```python
from build123d import *

# Parameters (mm, degrees)
BOSS_EXTRU_1_CONTOUR_CRAN_DEPTH              = 1.6
ENTRETOISES_R                                = 2
BOSS_EXTRU_1_ENTRETOISES_DEPTH               = 4.6
TROUS_VIS_M2_R                               = 1
ENL_V_MAT_EXTRU_1_TROUS_VIS_M2_DEPTH         = 4.6
CONNECTEURS_BLANCS_W                         = 15
CONNECTEURS_BLANCS_H                         = 4.3
CONNECTEURS_BLANCS_W_2                       = 10
BOSS_EXTRU_2_CONNECTEURS_BLANCS_DEPTH        = 3.7
OUVERTURE_GROS_CONNECTEUR_BLANC_W            = 14
OUVERTURE_GROS_CONNECTEUR_BLANC_H            = 2.7
ENL_V_MAT_EXTRU_2_OUVERTURE_GROS_CONNE_DEPTH = 3.7
OUVERTURE_PETIT_CONNECTEUR_BLANC_W           = 9
OUVERTURE_PETIT_CONNECTEUR_BLANC_H           = 2.7
ENL_V_MAT_EXTRU_3_OUVERTURE_PETIT_CONN_DEPTH = 3.7


with BuildPart() as part:
    # Contour_Écran → Boss.-Extru.1_Contour_Écran (new body)
    with BuildSketch(Plane.XY):
        with BuildLine():
            Line((-6.5, -20.3), (6.5, -20.3))
            ThreePointArc((6.5, -20.3), (7.668481961, -17.144005216), (10.005084126, -14.722034222))
            ThreePointArc((10.005084126, -14.722034222), (0, 17.8), (-10.005084126, -14.722034222))
            ThreePointArc((-10.005084126, -14.722034222), (-7.668481961, -17.144005216), (-6.5, -20.3))
        make_face()
    extrude(amount=BOSS_EXTRU_1_CONTOUR_CRAN_DEPTH)

    # Entretoises → Boss.-Extru.1_Entretoises (add)
    with BuildSketch(Plane(origin=(0, 0, 0), x_dir=(-1, 0, 0), z_dir=(0, 0, -1))):
        with Locations((-12.5, 9.5)):
            Circle(ENTRETOISES_R)
        with Locations((12.5, 9.5)):
            Circle(ENTRETOISES_R)
        with Locations((12.5, -9.5)):
            Circle(ENTRETOISES_R)
        with Locations((-12.5, -9.5)):
            Circle(ENTRETOISES_R)
    extrude(amount=BOSS_EXTRU_1_ENTRETOISES_DEPTH)

    # Trous_Vis_M2 → Enlèv. mat.-Extru.1_Trous_Vis_M2 (cut)
    with BuildSketch(Plane(origin=(0, 0, -4.6), x_dir=(-1, 0, 0), z_dir=(0, 0, -1))):
        with Locations((-12.5, 9.5)):
            Circle(TROUS_VIS_M2_R)
        with Locations((12.5, 9.5)):
            Circle(TROUS_VIS_M2_R)
        with Locations((12.5, -9.5)):
            Circle(TROUS_VIS_M2_R)
        with Locations((-12.5, -9.5)):
            Circle(TROUS_VIS_M2_R)
    extrude(amount=-ENL_V_MAT_EXTRU_1_TROUS_VIS_M2_DEPTH, mode=Mode.SUBTRACT)

    # Connecteurs_Blancs → Boss.-Extru.2_Connecteurs_Blancs (add)
    with BuildSketch(Plane(origin=(0, 0, 0), x_dir=(-1, 0, 0), z_dir=(0, 0, -1))):
        with Locations((0, 12.65)):
            Rectangle(CONNECTEURS_BLANCS_W, CONNECTEURS_BLANCS_H)
        with Locations((0, -6.15)):
            Rectangle(CONNECTEURS_BLANCS_W_2, CONNECTEURS_BLANCS_H)
    extrude(amount=BOSS_EXTRU_2_CONNECTEURS_BLANCS_DEPTH)

    # Ouverture_gros_connecteur_blanc → Enlèv. mat.-Extru.2_Ouverture_gros_connecteur_blanc (cut)
    with BuildSketch(Plane(origin=(0, 14.8, 0), x_dir=(1, 0, 0), z_dir=(0, 1, 0))):
        with Locations((0, 1.85)):
            Rectangle(OUVERTURE_GROS_CONNECTEUR_BLANC_W, OUVERTURE_GROS_CONNECTEUR_BLANC_H)
    extrude(amount=-ENL_V_MAT_EXTRU_2_OUVERTURE_GROS_CONNE_DEPTH, mode=Mode.SUBTRACT)

    # Ouverture_petit_connecteur_blanc → Enlèv. mat.-Extru.3_Ouverture_petit_connecteur_blanc (cut)
    with BuildSketch(Plane(origin=(0, -4, 0), x_dir=(1, 0, 0), z_dir=(0, 1, 0))):
        with Locations((0, 1.85)):
            Rectangle(OUVERTURE_PETIT_CONNECTEUR_BLANC_W, OUVERTURE_PETIT_CONNECTEUR_BLANC_H)
    extrude(amount=-ENL_V_MAT_EXTRU_3_OUVERTURE_PETIT_CONN_DEPTH, mode=Mode.SUBTRACT)


solid = part.part
```
The listing builds one solid part. Answer for the finished solid, in the listing's coordinates (mm). A direction names the side the tool comes from. Give positions to 0.01 mm unless a question says otherwise; leave off trailing zeros. Order: outer loops, then holes, each group sorted by start corner. A loop starts at its lowest first (then second) coordinate and runs counter-clockwise, first axis right, second up.
Item 1: Find the intervals of material crossed by probe 1 along Y at (x, z) = (-12.5, -2); probe 2 along Z at (x, y) = (10, -8); probe 3 along X at (y, z) = (8, -2.5), in increasing order.
From the geometry:
probe 1: y = -11.5 to -10.5, -8.5 to -7.5, 7.5 to 8.5, 10.5 to 11.5
probe 2: z = 0 to 1.6
probe 3: x = -13.82 to -11.18, 11.18 to 13.82
Item 2: Which of the six approach directions +Z, -Z, +X, -X, +Y, -Y give full straight-line access (tool end or side, diameter ignored) to faces 4 (the face through (-5, -6, -2)), 5 (the face through (0, 13, -3.2)), 6 (the face through (-12, -9, 0)), 7 (the face through (-7.5, 13, -2)), 8 (the face through (-0.3, -4, -0.3))?
From the geometry:
face 4: -Z, -Y
face 5: +Y
face 6: -Z
face 7: -Z, +Y, -Y
face 8: -Z, +X, -X
Item 3: The part is cut by section A-A, the plane z = -2.5. Count the separate pieces of the cut face and the enclosed holes in it, and give its area (3 significant figures).
From the geometry:
separate pieces: 6
enclosed holes: 4
area: 60.1 mm2
Item 4: The part is cut by section C-C, the plane y = -10. Give the vertices of the cut face in (x, z).
From the geometry:
outline: (-14.73, 0) - (-14.44, 0) - (-14.44, -4.6) - (-13.37, -4.6) - (-13.37, 0) - (-11.63, 0) - (-11.63, -4.6) - (-10.56, -4.6) - (-10.56, 0) - (10.56, 0) - (10.56, -4.6) - (11.63, -4.6) - (11.63, 0) - (13.37, 0) - (13.37, -4.6) - (14.44, -4.6) - (14.44, 0) - (14.73, 0) - (14.73, 1.6) - (-14.73, 1.6) - close
Item 5: The part is cut by section B-B, the plane x = 0. Give the vertices of the cut face in (y, z).
From the geometry:
outline: (-20.3, 0) - (-8.3, 0) - (-8.3, -3.7) - (-4, -3.7) - (-4, -3.2) - (-7.7, -3.2) - (-7.7, -0.5) - (-4, -0.5) - (-4, 0) - (10.5, 0) - (10.5, -3.7) - (14.8, -3.7) - (14.8, -3.2) - (11.1, -3.2) - (11.1, -0.5) - (14.8, -0.5) - (14.8, 0) - (17.8, 0) - (17.8, 1.6) - (-20.3, 1.6) - close
Item 6: The part is cut by section D-D, the plane y = -5. Give the vertices of the cut face in (x, z).
From the geometry:
outline: (-17.08, 0) - (-5, 0) - (-5, -3.7) - (5, -3.7) - (5, 0) - (17.08, 0) - (17.08, 1.6) - (-17.08, 1.6) - close; hole (-4.5, -3.2) - (4.5, -3.2) - (4.5, -0.5) - (-4.5, -0.5) - close
Item 7: For a pull along Y with two mould halves and no side action, classify faces 1 (the face through (0, -8.3, -2)), 2 (the face through (4.5, -6, -2)), 3 (the face through (-7, 13, -2)) as pulls with the +Y half, pulls with the -Y half, needs draft (parallel to the pull), parting line crosses it, or undercut.
From the geometry:
face 1: pulls with the -Y half
face 2: undercut
face 3: needs draft
Item 8: Given pin 1 Ø1.1 at (x, y) = (1, 13) entering from -Z; pin 2 Ø0.8 at (y, z) = (12, -1.5) entering from +X; pin 3 Ø2.5 at (x, y) = (12.5, 9.5) entering from -Z; pin 4 Ø1.1 at (y, z) = (13, -2.5) entering from -X, each flat-ended and moving along its own axis, determine where each tip first touches the part or whether it passes through.
From the geometry:
pin 1: stops at z = -3.7
pin 2: stops at x = 7.5
pin 3: stops at z = -4.6
pin 4: stops at x = -7.5
